Work out the finished part from the listing and answer in its coordinate system (mm). A direction names the side the tool comes from. Coordinates: 2 decimals unless noted, no trailing zeros. Write each loop counter-clockwise with the first axis right and the second up, starting at its lowest first coordinate (ties: lowest second). Pieces come first, ordered by that corner, then holes. Notation, with made-up numbers: (-16, 59.25) - (-1, 59.25) arc R38 cw to (-1, 97.25) - close; hole circle Ø11 at (-1.75, -28.75). An arc over 180 degrees is marked (long way). One line per item, written item: value.
```python
from build123d import *

# Parameters (mm, degrees)
F0_W     = 83.5
F0_H     = 55
F1_DEPTH = 70
F2_W     = 43.5
F2_H     = 20.677742
F3_DEPTH = 70.001
F5_DEPTH = 55.001


with BuildPart() as f1:
    # F0 (on Front) → F1 (new body)
    with BuildSketch(Plane.XZ):
        with Locations((41.75, 27.5)):
            Rectangle(F0_W, F0_H)
    extrude(amount=F1_DEPTH)

    # F2 (on Front) → F3 (cut, through all)
    with BuildSketch(Plane.XZ):
        with Locations((41.75, 44.661129)):
            Rectangle(F2_W, F2_H)
    extrude(amount=F3_DEPTH, mode=Mode.SUBTRACT)

    # F4 (on Top) → F5 (cut, through all)
    with BuildSketch(Plane.XY):
        Polygon((33.5, -54.897401), (0, -54.897401), (0, -70), (70, -70), (70, -51.566027), (53.5, -51.566027), (53.5, -40.276553), (33.5, -40.276553), align=None)
    extrude(amount=F5_DEPTH, mode=Mode.SUBTRACT)


solid = f1.part
```
Item 1: Section A-A, the plane z = 38 is taken. Determine the outline of the cut face in (x, y), then the cut area to 3 significant figures.
Evaluation:
outline: (0, -54.9) - (20, -54.9) - (20, 0) - (0, 0) - close; (63.5, -51.57) - (70, -51.57) - (70, -70) - (83.5, -70) - (83.5, 0) - (63.5, 0) - close
area: 2,380 mm2
Item 2: Given pin 1 (10 mm diameter, centred on x = 39, z = 22, fed in from -Y); pin 2 (9 mm diameter, centred on y = -64.5, z = 22.5, fed in from -X); pin 3 (8 mm diameter, centred on x = 62.5, z = 28, fed in from -Y), each flat-ended and moving along its own axis, determine where each tip first touches the part or whether it passes through.
Evaluation:
pin 1: stops at y = -40.28
pin 2: stops at x = 70
pin 3: stops at y = -51.57
Item 3: Which of the six approach directions +Z, -Z, +X, -X, +Y, -Y give full straight-line access (tool end or side, diameter ignored) to faces 1 (the face through (41, 0, 22)), 2 (the face through (70, -61, 27)), 3 (the face through (41, -27, 34.322)), 4 (the face through (17, -54.897, 21))?
Evaluation:
face 1: +Z, -Z, +X, -X, +Y
face 2: +Z, -Z, -Y
face 3: +Z, +Y, -Y
face 4: +Z, -Z, -X, -Y
Item 4: Section D-D, the plane x = 38 is taken. Determine the outline of the cut face in (y, z).
Evaluation:
outline: (-40.28, 0) - (0, 0) - (0, 34.32) - (-40.28, 34.32) - close
Item 5: Determine the mould class of faces 5 (the face through (33.5, -47, 17)), 6 (the face through (83.5, -35, 27)), 7 (the face through (0, -27, 27)), 8 (the face through (10, -27, 55)) for opening direction X: +X half, -X half, draft (parallel to the pull), parting line (faces both ways), or undercut.
Evaluation:
face 5: undercut
face 6: +X half
face 7: -X half
face 8: draft
Item 6: Section B-B, the plane y = -16.5 is taken. Determine the outline of the cut face in (x, z).
Evaluation:
outline: (0, 0) - (83.5, 0) - (83.5, 55) - (63.5, 55) - (63.5, 34.32) - (20, 34.32) - (20, 55) - (0, 55) - close
Item 7: Consider probe 1 along X at (y, z) = (-47, 12); probe 2 along X at (y, z) = (-20, 44); probe 3 along Y at (x, z) = (27.5, 8.5). Determine where each line is inside the solid, lowest interval first.
Evaluation:
probe 1: x = 0 to 33.5, 53.5 to 83.5
probe 2: x = 0 to 20, 63.5 to 83.5
probe 3: y = -54.9 to 0
Item 8: Section C-C, the plane z = 8.5 is taken. Determine the outline of the cut face in (x, y).
Evaluation:
outline: (0, -54.9) - (33.5, -54.9) - (33.5, -40.28) - (53.5, -40.28) - (53.5, -51.57) - (70, -51.57) - (70, -70) - (83.5, -70) - (83.5, 0) - (0, 0) - close
